from build123d import *

# Parameters (mm, degrees)
SKETCH1_R                        = 0.5
BOSS_EXTRUDE1_DEPTH              = 13.9
F_0_4_0_4_DIAMETER_HOLE1_D       = 0.4
F_0_75_0_75_DIAMETER_HOLE2_D     = 0.75
F_0_75_0_75_DIAMETER_HOLE2_DEPTH = 11.325
F_0_75_0_75_DIAMETER_HOLE2_TIP   = 0.225322732
F_0_6_0_6_DIAMETER_HOLE4_D       = 0.6
F_0_6_0_6_DIAMETER_HOLE4_DEPTH   = 2.425
F_0_6_0_6_DIAMETER_HOLE4_TIP     = 0.180258186


with BuildPart() as part:
    # Sketch1 → Boss-Extrude1 (new body)
    with BuildSketch(Plane(origin=(0, 0, 0), x_dir=(1, 0, 0), z_dir=(0, 1, 0))):
        with Locations(Location((0, 0, 0), (0, 0, 270))):
            Circle(SKETCH1_R)
    extrude(amount=BOSS_EXTRUDE1_DEPTH)

    # Ø0.4 (0.4) Diameter Hole1 (through all)
    with Locations(Plane(origin=(0, 13.9, 0), x_dir=(-1, 0, 0), z_dir=(0, 1, 0))):
        with Locations((0, 0)):
            Hole(F_0_4_0_4_DIAMETER_HOLE1_D / 2)

    # Ø0.75 (0.75) Diameter Hole2
    with Locations(Plane(origin=(0, 13.9, 0), x_dir=(-1, 0, 0), z_dir=(0, 1, 0))):
        with Locations((0, 0)):
            Hole(F_0_75_0_75_DIAMETER_HOLE2_D / 2, depth=F_0_75_0_75_DIAMETER_HOLE2_DEPTH)
            with Locations((0, 0, -(F_0_75_0_75_DIAMETER_HOLE2_DEPTH + F_0_75_0_75_DIAMETER_HOLE2_TIP / 2))):  # 118° drill point
                Cone(0, F_0_75_0_75_DIAMETER_HOLE2_D / 2, F_0_75_0_75_DIAMETER_HOLE2_TIP, mode=Mode.SUBTRACT)

    # Ø0.6 (0.6) Diameter Hole4
    with Locations(Plane.XZ):
        with Locations((0, 0)):
            Hole(F_0_6_0_6_DIAMETER_HOLE4_D / 2, depth=F_0_6_0_6_DIAMETER_HOLE4_DEPTH)
            with Locations((0, 0, -(F_0_6_0_6_DIAMETER_HOLE4_DEPTH + F_0_6_0_6_DIAMETER_HOLE4_TIP / 2))):  # 118° drill point
                Cone(0, F_0_6_0_6_DIAMETER_HOLE4_D / 2, F_0_6_0_6_DIAMETER_HOLE4_TIP, mode=Mode.SUBTRACT)


solid = part.part
Design review of the part built by this model. Coordinates are the model's own, in mm. Round coordinates to 2 decimals unless told otherwise and drop trailing zeros. Write each loop counter-clockwise with the first axis right and the second up, starting at its lowest first coordinate (ties: lowest second). Pieces come first, ordered by that corner, then holes.
Item 1: Consider section D-D on y = 8. Give the boundary of the cut face in (x, z) (3 decimals), and give its area (3 significant figures).
Item 2: Consider section B-B on x = 0. Give the boundary of the cut face in (y, z) (3 decimals), and give its area (3 significant figures).
Item 3: Wall thickness on L1, parallel to X at y = 0.9, z = 0; L2, parallel to X at y = 9.5, z = -0.3 (3 decimals): over which ranges is each line inside the solid? List them lowest first.
Item 4: Consider section C-C on y = 1. Give the boundary of the cut face in (x, z), and give its area (3 significant figures).
Item 5: Consider section A-A on z = 0. Give the boundary of the cut face in (x, y) (3 decimals).
Check values:
1. outline: circle Ø1 at (0, 0); hole circle Ø0.75 at (0, 0)
1. area: 0.344 mm2
2. outline: (0, -0.5) - (13.9, -0.5) - (13.9, -0.375) - (2.575, -0.375) - (2.477, -0.213) - (2.425, -0.3) - (0, -0.3) - close; (0, 0.3) - (2.425, 0.3) - (2.477, 0.213) - (2.575, 0.375) - (13.9, 0.375) - (13.9, 0.5) - (0, 0.5) - close
2. area: 3.87 mm2
3. L1: x = -0.5 to -0.3, 0.3 to 0.5
3. L2: x = -0.4 to -0.225, 0.225 to 0.4
4. outline: circle Ø1 at (0, 0); hole circle Ø0.6 at (0, 0)
4. area: 0.503 mm2
5. outline: (-0.5, 0) - (-0.3, 0) - (-0.3, 2.425) - (-0.213, 2.477) - (-0.375, 2.575) - (-0.375, 13.9) - (-0.5, 13.9) - close; (0.213, 2.477) - (0.3, 2.425) - (0.3, 0) - (0.5, 0) - (0.5, 13.9) - (0.375, 13.9) - (0.375, 2.575) - close
